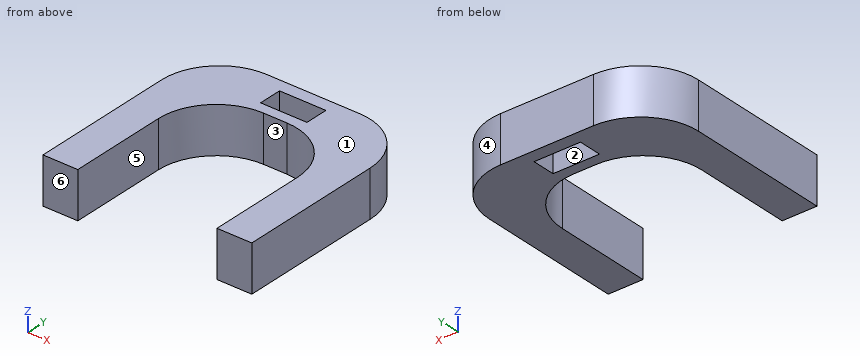
from build123d import *

# Parameters (mm, degrees)
SKETCH_2_W          = 18
SKETCH_2_H          = 21.5
EXTRUDE_1_DEPTH     = 4
SKETCH_3_W          = 12
SKETCH_3_H          = 17.5
CUT_EXTRUDE_1_DEPTH = 29.324018077
FILLET_1_R          = 5
FILLET_2_R          = 5
SKETCH_4_W          = 4
SKETCH_4_H          = 2
CUT_EXTRUDE_2_DEPTH = 29.324018077
SKETCH_8_W          = 3
SKETCH_8_H          = 4
CUT_EXTRUDE_5_DEPTH = 29.324018077


with BuildPart() as part:
    # ｽｹｯﾁ2 → ﾎﾞｽ - 押し出し1 (new body)
    with BuildSketch(Plane.XY):
        with Locations((9, 10.75)):
            Rectangle(SKETCH_2_W, SKETCH_2_H)
    extrude(amount=EXTRUDE_1_DEPTH)

    # ｽｹｯﾁ3 → ｶｯﾄ - 押し出し1 (cut, through all)
    with BuildSketch(Plane.XY.offset(4)):
        with Locations((9, 8.75)):
            Rectangle(SKETCH_3_W, SKETCH_3_H)
    extrude(amount=-CUT_EXTRUDE_1_DEPTH, mode=Mode.SUBTRACT)

    # ﾌｨﾚｯﾄ1
    fillet_1_edges = [part.edges().sort_by_distance(p)[0] for p in [
        (3, 17.5, 2),
        (15, 17.5, 2),
    ]]
    fillet(fillet_1_edges, radius=FILLET_1_R)

    # ﾌｨﾚｯﾄ2
    fillet_2_edges = [part.edges().sort_by_distance(p)[0] for p in [
        (0, 21.5, 2),
        (18, 21.5, 2),
    ]]
    fillet(fillet_2_edges, radius=FILLET_2_R)

    # ｽｹｯﾁ4 → ｶｯﾄ - 押し出し2 (cut, through all)
    with BuildSketch(Plane.XY.offset(4)):
        with Locations((9, 19.400947982)):
            Rectangle(SKETCH_4_W, SKETCH_4_H)
    extrude(amount=-CUT_EXTRUDE_2_DEPTH, mode=Mode.SUBTRACT)

    # ｽｹｯﾁ8 → ｶｯﾄ - 押し出し5 (cut, through all)
    with BuildSketch(Plane.XY.offset(4)):
        with Locations((1.5, 2)):
            Rectangle(SKETCH_8_W, SKETCH_8_H)
        with Locations((16.5, 2)):
            Rectangle(SKETCH_8_W, SKETCH_8_H)
    extrude(amount=-CUT_EXTRUDE_5_DEPTH, mode=Mode.SUBTRACT)


solid = part.part
The listing builds one solid part. Answer for the finished solid, in the listing's coordinates (mm). Face numbers are marked on the shaded views. A direction names the side the tool comes from. Round coordinates to 2 decimals unless told otherwise and drop trailing zeros. Order: outer loops, then holes, each group sorted by start corner. A loop starts at its lowest first (then second) coordinate and runs counter-clockwise, first axis right, second up. Notation, with made-up numbers: (15, 68.25) - (42, 68.25) arc R21 ccw to (42, 104.25) - close; hole circle Ø9 at (59, 87). An arc over 180 degrees is marked (long way). Write item = value, one per line. Start each with the question number.
1) Section A-A, the plane x = 9.5 is taken. Write down the section's boundary in (y, z).
2) Section B-B, the plane y = 11.25 is taken. Write down the section's boundary in (x, z), plus the area to 3 significant figures.
3) Section C-C, the plane z = 0.65 is taken. Write down the section's boundary in (x, y), plus the area to 3 significant figures.
4) Section D-D, the plane x = 17 is taken. Write down the section's boundary in (y, z).
5) For the marked faces 1, 2 and 3, determine the directions among +Z, -Z, +X, -X, +Y, -Y from which every point of the face is accessible in a straight line to the end or side of a thin tool.
6) For a pull along X with two mould halves and no side action, classify the marked faces 4, 5 and 6 as released by +X, released by -X, zero draft, split by the parting line, or undercut.
7) Straight lines are drawn through the part: L1, parallel to X at y = 8.25, z = 2.9; L2, parallel to Y at x = 9.5, z = 2.25; L3, parallel to X at y = 14.5, z = 3.1. For each, find the intervals that lie inside material, in ascending order.
8) Given pin 1 (2 mm diameter, centred on y = 19.5, z = 2.5, fed in from +X); pin 2 (1.2 mm diameter, centred on x = 8, z = 2.5, fed in from -Y); pin 3 (2 mm diameter, centred on y = 20, z = 2.5, fed in from -X), each flat-ended and moving along its own axis, determine where each tip first touches the part or whether it passes through.
Results list:
q1.outline = (17.5, 0) - (18.4, 0) - (18.4, 4) - (17.5, 4) - close; (20.4, 0) - (21.5, 0) - (21.5, 4) - (20.4, 4) - close
q2.outline = (0, 0) - (3, 0) - (3, 4) - (0, 4) - close; (15, 0) - (18, 0) - (18, 4) - (15, 4) - close
q2.area = 24.0 mm^2
q3.outline = (0, 4) - (3, 4) - (3, 12.5) arc R5 cw to (8, 17.5) - (10, 17.5) arc R5 cw to (15, 12.5) - (15, 4) - (18, 4) - (18, 16.5) arc R5 ccw to (13, 21.5) - (5, 21.5) arc R5 ccw to (0, 16.5) - close; hole (7, 18.4) - (11, 18.4) - (11, 20.4) - (7, 20.4) - close
q3.area = 145 mm^2
q4.outline = (4, 0) - (19.5, 0) - (19.5, 4) - (4, 4) - close
q5.face_1 = +Z, +X, -X, +Y, -Y
q5.face_2 = +Z, -Z
q5.face_3 = +Z, -Z, -Y
q6.face_4 = released by +X
q6.face_5 = undercut
q6.face_6 = zero draft
q7.L1 = 0 to 3, 15 to 18
q7.L2 = 17.5 to 18.4, 20.4 to 21.5
q7.L3 = 0 to 3.42, 14.58 to 18
q8.pin_1 = 17.58
q8.pin_2 = 17.46
q8.pin_3 = 0.67
